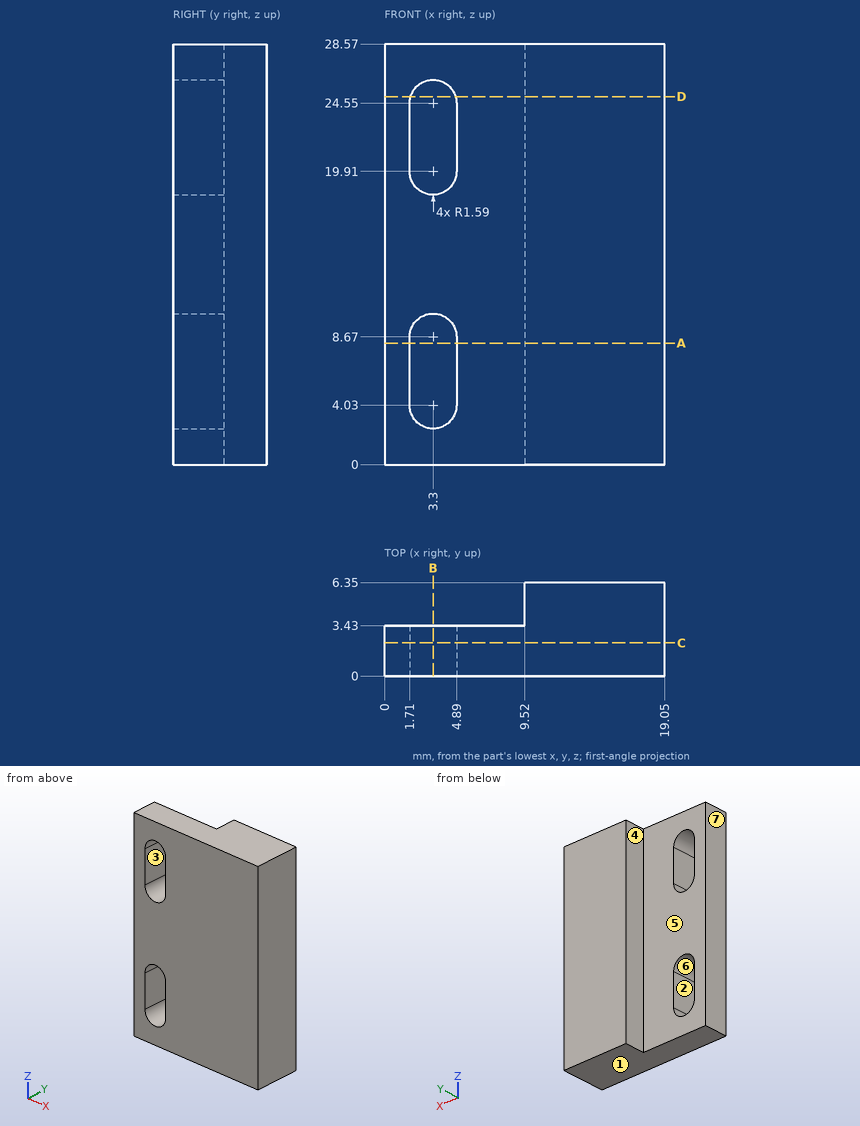
Geometry: see drawing. Coordinates: mm, zero at the bounding-box minimum. A direction names the side the tool comes from. Coordinates: 2 decimals unless noted, no trailing zeros. Order: outer loops, then holes, each group sorted by start corner. A loop starts at its lowest first (then second) coordinate and runs counter-clockwise, first axis right, second up. Notation, with made-up numbers: M 42,83 L 78,83 A14 cw 78,110 Z; hole C -28,8.25 d3. An arc over 180 degrees is marked long. Write each question's results on one line, items separated by ' | '. Start each with the question number.
1) Draft query along Z for the marked faces 1, 2, 3 and 4. Return one class per face: released by +Z, released by -Z, zero draft, split by the parting line, or undercut.
2) Contact query for flat-ended pins moving along their axis: pin 1 Ø3 at (x, z) = (2.5, 9.5) entering from +Y; pin 2 Ø1 at (x, z) = (7.5, 13) entering from -Y. Output: stop coordinate, or through.
3) Access query for the marked faces 5, 6 and 7. Directions: +Z, -Z, +X, -X, +Y, -Y. A direction counts if a zero-diameter tool reaches every point of the face in a straight line with its end or side. Return the directions, or none.
4) Line query: line 1 (Z direction, x = 4, y = 1.5); line 2 (X direction, y = 1, z = 22.75); line 3 (Y direction, x = 1, z = 4.5). Output: solid intervals per line, ascending. Write a range as from..to.
5) Section query A-A (z = 8.25). Return the cut outline in (x, y).
6) Section query C-C (y = 2.25). Return the cut outline in (x, z), plus the area to 3 significant figures.
7) Section query D-D (z = 25). Return the cut outline in (x, y) (3 decimals), plus the area to 3 significant figures.
8) Section query B-B (x = 3.3). Return the cut outline in (y, z).
Answers:
1) face 1: released by -Z | face 2: undercut | face 3: undercut | face 4: zero draft
2) pin 1: stops at y = 3.43 | pin 2: stops at y = 0
3) face 5: +Z, -Z, -X, +Y | face 6: +Y, -Y | face 7: +Z, -Z, -X, +Y, -Y
4) line 1: z = 0..2.6, 10.1..18.48, 25.98..28.57 | line 2: x = 0..1.71, 4.89..19.05 | line 3: y = 0..3.43
5) outline: M 0,0 L 1.71,0 L 1.71,3.43 L 0,3.43 Z; M 4.89,0 L 19.05,0 L 19.05,6.35 L 9.52,6.35 L 9.52,3.43 L 4.89,3.43 Z
6) outline: M 0,0 L 19.05,0 L 19.05,28.57 L 0,28.57 Z; hole M 1.71,4.03 A1.59 ccw 4.89,4.03 L 4.89,8.67 A1.59 ccw 1.71,8.67 Z; hole M 1.71,19.91 A1.59 ccw 4.89,19.91 L 4.89,24.55 A1.59 ccw 1.71,24.55 Z | area: 499 mm^2
7) outline: M 0,0 L 1.775,0 L 1.775,3.43 L 0,3.43 Z; M 4.825,0 L 19.05,0 L 19.05,6.35 L 9.52,6.35 L 9.52,3.43 L 4.825,3.43 Z | area: 82.7 mm^2
8) outline: M 0,0 L 3.43,0 L 3.43,2.44 L 0,2.44 Z; M 0,10.26 L 3.43,10.26 L 3.43,18.32 L 0,18.32 Z; M 0,26.14 L 3.43,26.14 L 3.43,28.57 L 0,28.57 Z
